Geometry: final body of the model. Coordinates: model frame, mm. Give positions to 0.01 mm unless a question says otherwise; leave off trailing zeros. Order: outer loops, then holes, each group sorted by start corner. A loop starts at its lowest first (then second) coordinate and runs counter-clockwise, first axis right, second up. Notation, with made-up numbers: M -31.5,18.5 L -3.5,18.5 A20 ccw -3.5,42.5 Z; hole C 5,-6.75 d11. An arc over 180 degrees is marked long. Use CSV: the item, a comma, the result in double quotes.
Autodesk Inventor part; units mm, degrees
ref_plane "YZ Plane" through (0, 0, 0) normal (1, 0, 0) x (0, 1, 0)
ref_plane "XZ Plane" through (0, 0, 0) normal (0, 1, 0) x (-1, 0, 0)
ref_plane "XY Plane" through (0, 0, 0) normal (0, 0, 1) x (1, 0, 0)
sketch "Sketch1" plane through (0, 0, 0) normal (0, 0, 1) x (1, 0, 0)
  circle A0 centre (0, 0) radius 14.2875
  circle A1 centre (0, 0) radius 20.32 construction
  circle A2 centre (0, 50.8) radius 30.48 construction
  circle A3 centre (0, 50.8) radius 14.2875
  circle A4 centre (0, 50.8) radius 35.56 construction
  line L0 (0, 81.28) -> (0, 86.36)
  circle A5 centre (0, 0) radius 25.4 construction
  line L1 (0, 20.32) -> (0, 25.4) construction
  circle A6 centre (-31.7808, 17.1604) radius 6.35 construction
  circle A7 centre (31.1821, 16.6047) radius 6.35 construction
  line L2 (-27.42, 21.7763) -> (-24.4204, 24.9513) construction
  line L3 (-26.1933, 14.1434) -> (-22.3499, 12.0681) construction
  line L4 (26.8213, 11.9889) -> (23.8217, 8.8139) construction
  line L5 (26.9034, 21.2968) -> (23.9604, 24.5243) construction
  circle A8 centre (-31.7808, 17.1604) radius 3.2639
  circle A9 centre (31.1821, 16.6047) radius 3.2639
  line L6 (-37.2911, 14.0047) -> (-22.0413, -12.6231)
  line L7 (36.718, 13.494) -> (22.1435, -12.4429)
  line L8 (-38.1134, 17.6293) -> (-35.4629, 53.4258)
  line L9 (37.522, 16.9618) -> (35.5037, 52.7995)
  arc A10 (-38.1134, 17.6293) -> (-37.2911, 14.0047) centre (-31.7808, 17.1604) ccw
  arc A11 (36.718, 13.494) -> (37.522, 16.9618) centre (31.1821, 16.6047) ccw
  arc A12 (35.5037, 52.7995) -> (-35.4629, 53.4258) centre (0, 50.8) ccw
  arc A13 (-22.0413, -12.6231) -> (22.1435, -12.4429) centre (0, 0) ccw
  dimension "d1" = 40.64
  dimension "d0" = 28.575
  dimension "d2" = 60.96
  dimension "d3" = 28.575
  dimension "d4" = 5.08
  dimension "d5" = 71.12
  dimension "d6" = 5.08
  dimension "d9" = 12.7
  dimension "d10" = 3.175
  dimension "d11" = 6.5278
  dimension "d12" = 6.5278
extrude "Extrusion2" add sketch "Sketch1" along normal blind 6.35
properties part number "BottomPlate" material "Aluminum 6061"
1. Section A-A, the plane x = 8. Return the cut outline in (y, z), plus the area to 3 significant figures.
Answer:
outline,"M -24.11,0 L -11.84,0 L -11.84,6.35 L -24.11,6.35 Z; M 11.84,0 L 38.96,0 L 38.96,6.35 L 11.84,6.35 Z; M 62.64,0 L 85.45,0 L 85.45,6.35 L 62.64,6.35 Z"
area,"395 mm2"
2. Pin query (flat end, axial travel): pin 1 Ø1 at (y, z) = (60, 5) entering from -X; pin 2 Ø1 at (y, z) = (37, 3.5) entering from +X. Return the tip coordinate at first contact, or that it passes through.
Answer:
pin 1,"x = -34.48"
pin 2,"x = 36.42"
3. Section B-B, the plane z = 5. Return the cut outline in (x, y) (1 decimal).
Answer:
outline,"M -38.1,17.6 A6.4 ccw -37.3,14 L -22,-12.6 A25.4 ccw 22.1,-12.4 L 36.7,13.5 A6.3 ccw 37.5,17 L 35.5,52.8 A35.6 ccw -35.5,53.4 Z; hole C -31.8,17.2 d6.5; hole C 0,0 d28.6; hole C 0,50.8 d28.6; hole C 31.2,16.6 d6.5"
4. Pull-direction query (X, two-part tool) for faces 1 (the face through (29.533, 0.707, 3.131)), 2 (the face through (-1.86, 36.634, 3.131)), 3 (the face through (-36.807, 35.277, 3.131)); classes: +X half, -X half, draft (parallel to the pull), parting line (faces both ways), or undercut.
Answer:
face 1,"+X half"
face 2,"undercut"
face 3,"-X half"
5. Section D-D, the plane x = 29.5. Return the cut outline in (y, z).
Answer:
outline,"M 0.65,0 L 13.81,0 L 13.81,6.35 L 0.65,6.35 Z; M 19.4,0 L 70.66,0 L 70.66,6.35 L 19.4,6.35 Z"
6. Line query: line 1 (Y direction, x = 0.5, z = 4); line 2 (Y direction, x = -8, z = 2); line 3 (X direction, y = 19, z = 3). Output: solid intervals per line, ascending.
Answer:
line 1,"-25.4 to -14.28, 14.28 to 36.52, 65.08 to 86.36"
line 2,"-24.11 to -11.84, 11.84 to 38.96, 62.64 to 85.45"
line 3,"-38.01 to -34.48, -29.08 to 28.96, 33.4 to 37.41"
7. Section C-C, the plane y = 50.8. Return the cut outline in (x, z), plus the area to 3 significant figures.
Answer:
outline,"M -35.66,0 L -14.29,0 L -14.29,6.35 L -35.66,6.35 Z; M 14.29,0 L 35.62,0 L 35.62,6.35 L 14.29,6.35 Z"
area,"271 mm2"
